Geometry check sheet. Reference: the model listing, model coordinates, mm. A direction names the side the tool comes from. Round coordinates to 2 decimals unless told otherwise and drop trailing zeros. Write each loop counter-clockwise with the first axis right and the second up, starting at its lowest first coordinate (ties: lowest second). Pieces come first, ordered by that corner, then holes.
from build123d import *

# Parameters (mm, degrees)
SKETCH_W             = 60
SKETCH_H             = 40
PAD_DEPTH            = 7
SKETCH001_R          = 3.5
POCKET_DEPTH         = 0.001
POCKET_DEPTH_BACK    = 7.001
SKETCH002_W          = 60
SKETCH002_H          = 5
PAD001_DEPTH         = 55
SKETCH003_W          = 60
SKETCH003_H          = 7
PAD002_DEPTH         = 15
SKETCH004_R          = 4
POCKET001_DEPTH      = 10
SKETCH005_R          = 15
POCKET002_DEPTH      = 10
SKETCH006_R          = 2
POCKET003_DEPTH      = 20.001
POCKET004_DEPTH      = 15
POCKET005_DEPTH      = 1
CHAMFER_SIZE         = 2.49
SKETCH009_W          = 5
SKETCH009_H          = 15
PAD003_DEPTH         = 48
POCKET006_DEPTH      = 62.001
POCKET006_DEPTH_BACK = 0.001
SKETCH011_W          = 30
SKETCH011_H          = 1.5
POCKET007_DEPTH      = 10
SKETCH013_R          = 1.25
POCKET008_DEPTH      = 40.001
SKETCH014_R          = 1.5
POCKET009_DEPTH      = 9.5


with BuildPart() as part:
    # Sketch → Pad (new body)
    with BuildSketch(Plane.XY):
        with Locations((5, 0)):
            Rectangle(SKETCH_W, SKETCH_H)
    extrude(amount=PAD_DEPTH)

    # Sketch001 → Pocket (cut, two sides)
    with BuildSketch(Plane.XY) as pocket_sk:
        with Locations((-11, 11)):
            Circle(SKETCH001_R)
        with Locations((-11, -11)):
            Circle(SKETCH001_R)
        with Locations((21, 11)):
            Circle(SKETCH001_R)
    extrude(amount=-POCKET_DEPTH, mode=Mode.SUBTRACT)
    extrude(pocket_sk.sketch, amount=POCKET_DEPTH_BACK, mode=Mode.SUBTRACT)

    # Sketch002 (on Face5 of Pocket) → Pad001 (join)
    with BuildSketch(Plane.XY.offset(7)):
        with Locations((5, -2.5)):
            Rectangle(SKETCH002_W, SKETCH002_H)
    extrude(amount=PAD001_DEPTH)

    # Sketch003 (on Face14 of Pad001) → Pad002 (join)
    with BuildSketch(Plane.XZ.offset(5)):
        with Locations((5, 58.5)):
            Rectangle(SKETCH003_W, SKETCH003_H)
    extrude(amount=PAD002_DEPTH)

    # Sketch004 (on Face20 of Pad002) → Pocket001 (cut)
    with BuildSketch(Plane.XY.offset(62)):
        with Locations((0, -10)):
            Circle(SKETCH004_R)
    extrude(amount=-POCKET001_DEPTH, mode=Mode.SUBTRACT)

    # Sketch005 (on Face13 of Pocket001) → Pocket002 (cut)
    with BuildSketch(Plane(origin=(0, 0, 0), x_dir=(-1, 0, 0), z_dir=(0, 1, 0))):
        with Locations((-7, 31)):
            Circle(SKETCH005_R)
    extrude(amount=-POCKET002_DEPTH, mode=Mode.SUBTRACT)

    # Sketch006 (on Face13 of Pocket002) → Pocket003 (cut, through all)
    with BuildSketch(Plane(origin=(0, 0, 0), x_dir=(-1, 0, 0), z_dir=(0, 1, 0))):
        with Locations((-22.5, 46.5)):
            Circle(SKETCH006_R)
        with Locations((8.5, 46.5)):
            Circle(SKETCH006_R)
        with Locations((-22.5, 15.5)):
            Circle(SKETCH006_R)
        with Locations((8.5, 15.5)):
            Circle(SKETCH006_R)
    extrude(amount=-POCKET003_DEPTH, mode=Mode.SUBTRACT)

    # Sketch007 (on Face5 of Pocket003) → Pocket004 (cut)
    with BuildSketch(Plane.XY.offset(7)):
        with BuildLine():
            ThreePointArc((-13.5, 14.5), (-17, 11), (-13.5, 7.5))
            Line((-13.5, 7.5), (-8.5, 7.5))
            ThreePointArc((-8.5, 7.5), (-5, 11), (-8.5, 14.5))
            Line((-13.5, 14.5), (-8.5, 14.5))
        make_face()
        with BuildLine():
            ThreePointArc((-13.5, -7.5), (-17, -11), (-13.5, -14.5))
            Line((-13.5, -14.5), (-8.5, -14.5))
            ThreePointArc((-8.5, -14.5), (-5, -11), (-8.5, -7.5))
            Line((-13.5, -7.5), (-8.5, -7.5))
        make_face()
        with BuildLine():
            ThreePointArc((24.5, 13.5), (21, 17), (17.5, 13.5))
            Line((17.5, 13.5), (17.5, 8.5))
            ThreePointArc((17.5, 8.5), (21, 5), (24.5, 8.5))
            Line((24.5, 13.5), (24.5, 8.5))
        make_face()
    extrude(amount=-POCKET004_DEPTH, mode=Mode.SUBTRACT)

    # Sketch008 (on Face5 of Pocket004) → Pocket005 (cut, symmetric)
    with BuildSketch(Plane.XY.offset(7)):
        with BuildLine():
            ThreePointArc((27.4, 13.5), (21, 19.9), (14.6, 13.5))
            Line((14.6, 13.5), (14.6, 8.5))
            ThreePointArc((14.6, 8.5), (21, 2.1), (27.4, 8.5))
            Line((27.4, 13.5), (27.4, 8.5))
        make_face()
        with BuildLine():
            ThreePointArc((-13.5, 17.4), (-19.9, 11), (-13.5, 4.6))
            Line((-13.5, 4.6), (-8.5, 4.6))
            ThreePointArc((-8.5, 4.6), (-2.1, 11), (-8.5, 17.4))
            Line((-13.5, 17.4), (-8.5, 17.4))
        make_face()
        with BuildLine():
            ThreePointArc((-13.5, -4.6), (-19.9, -11), (-13.5, -17.4))
            Line((-13.5, -17.4), (-8.5, -17.4))
            ThreePointArc((-8.5, -17.4), (-2.1, -11), (-8.5, -4.6))
            Line((-13.5, -4.6), (-8.5, -4.6))
        make_face()
    extrude(amount=POCKET005_DEPTH, both=True, mode=Mode.SUBTRACT)

    # Chamfer
    chamfer_edges = [part.edges().sort_by_distance(p)[0] for p in [
        (-17, 11, 6),
        (21, 5, 6),
        (-17, -11, 6),
    ]]
    chamfer(chamfer_edges, length=CHAMFER_SIZE)

    # Sketch009 (on Face37 of Chamfer) → Pad003 (join)
    with BuildSketch(Plane.XY.offset(7)):
        with Locations((32.5, -12.5)):
            Rectangle(SKETCH009_W, SKETCH009_H)
    extrude(amount=PAD003_DEPTH)

    # Sketch010 (on Face76 of Pad003) → Pocket006 (cut, two sides)
    with BuildSketch(Plane.XY.offset(62)) as pocket006_sk:
        with BuildLine():
            Line((-25, -20), (-25, -12))
            ThreePointArc((-25, -12), (-21.78316, -16.78316), (-17, -20))
            Line((-25, -20), (-17, -20))
        make_face()
    extrude(amount=-POCKET006_DEPTH, mode=Mode.SUBTRACT)
    extrude(pocket006_sk.sketch, amount=POCKET006_DEPTH_BACK, mode=Mode.SUBTRACT)

    # Sketch011 (on Face78 of Pocket006) → Pocket007 (cut)
    with BuildSketch(Plane.XY.offset(62)):
        with Locations((0, -10)):
            Rectangle(SKETCH011_W, SKETCH011_H)
    extrude(amount=-POCKET007_DEPTH, mode=Mode.SUBTRACT)

    # Sketch013 (on Face66 of Pocket007) → Pocket008 (cut, through all)
    with BuildSketch(Plane.XZ.offset(20)):
        with Locations((9, 51.5)):
            Circle(SKETCH013_R)
        with Locations((-9, 51.5)):
            Circle(SKETCH013_R)
    extrude(amount=-POCKET008_DEPTH, mode=Mode.SUBTRACT)

    # Sketch014 (on Face66 of Pocket008) → Pocket009 (cut)
    with BuildSketch(Plane.XZ.offset(20)):
        with Locations((-9, 58.5)):
            Circle(SKETCH014_R)
        with Locations((9, 58.5)):
            Circle(SKETCH014_R)
    extrude(amount=-POCKET009_DEPTH, mode=Mode.SUBTRACT)


solid = part.part
1. Section check C-C (z = 31). Record the cut outline in (x, y).
2. Section check D-D (x = 23.5). State how many separate pieces and enclosed holes the cut face has, plus the area to 3 significant figures.
3. Section check A-A (z = 51.5). Record the cut outline in (x, y).
4. Depth check by flat-ended pin: pin 1 Ø7.5 at (x, z) = (12, 59) entering from +Y; pin 2 Ø5 at (x, y) = (-10, 6.5) entering from +Z; pin 3 Ø12 at (x, y) = (-17, 1) entering from -Z; pin 4 Ø2 at (x, z) = (26, 31) entering from -Y. Enter the tip coordinate at first touch or a pass-through.
5. Scan lines: line 1 along Z through (x, y) = (9, -15); line 2 along X through (y, z) = (-2, 15); line 3 along Z through (x, y) = (22.5, -1.7). Record each from-to range of solid material in increasing order.
6. Access from +Z, -Z, +X, -X, +Y, -Y to the whole of each face (thin tool, end or side, straight path). Record for faces 1 (the face through (-10, -5, 31)), 2 (the face through (-9, -15, 60)), 3 (the face through (-5, -11, 2)), 4 (the face through (21.09, 17.43, 3.94)).
7. Section check B-B (y = 11). Record the cut outline in (x, z), plus the area to 3 significant figures.
8. Release check for a two-part mould opening along Y. For faces 5 (the face through (16.24, 11.04, 4.77)), 6 (the face through (21, 5, 2)), 7 (the face through (5, 0, 0)), 8 (the face through (4.6, 0, 46.3)) record: +Y half, -Y half, draft (parallel to the pull), parting line (faces both ways), or undercut.
Results below:
1. outline: (-25, -5) - (-8, -5) - (-8, 0) - (-25, 0) - close; (22, -5) - (30, -5) - (30, -20) - (35, -20) - (35, 0) - (22, 0) - close
2. separate pieces: 4
2. enclosed holes: 0
2. area: 541 mm2
3. outline: (-25, -5) - (-10.25, -5) - (-10.25, 0) - (-25, 0) - close; (-7.75, -5) - (7.75, -5) - (7.75, 0) - (-7.75, 0) - close; (10.25, -5) - (30, -5) - (30, -20) - (35, -20) - (35, 0) - (10.25, 0) - close
4. pin 1: stops at y = 0
4. pin 2: stops at z = 7
4. pin 3: stops at z = 0
4. pin 4: stops at y = -5
5. line 1: z = 0 to 7, 55 to 57, 60 to 62
5. line 2: x = -25 to -10.44, -6.56 to 20.56, 24.44 to 35
5. line 3: z = 0 to 13.5, 17.5 to 44.5, 48.5 to 62
6. face 1: -X, -Y
6. face 2: -Y
6. face 3: -Z
6. face 4: +Z
7. outline: (-25, 0) - (-17, 0) - (-17, 3.51) - (-19.49, 6) - (-19.9, 6) - (-19.9, 7) - (-25, 7) - close; (-5, 0) - (17.5, 0) - (17.5, 3.51) - (15.01, 6) - (14.6, 6) - (14.6, 7) - (-2.1, 7) - (-2.1, 6) - (-2.51, 6) - (-5, 3.51) - close; (24.5, 0) - (35, 0) - (35, 7) - (27.4, 7) - (27.4, 6) - (26.99, 6) - (24.5, 3.51) - close
7. area: 263 mm2
8. face 5: undercut
8. face 6: undercut
8. face 7: draft
8. face 8: +Y half
